The model under review builds one solid part; all positions refer to its coordinate system, in mm. A direction names the side the tool comes from. Round coordinates to 2 decimals unless told otherwise and drop trailing zeros. Write each loop counter-clockwise with the first axis right and the second up, starting at its lowest first coordinate (ties: lowest second). Pieces come first, ordered by that corner, then holes. Notation, with made-up numbers: (42, 68) -> (53, 68) arc R19 cw to (53, 76) -> close; hole circle Ø7 at (-16, -32). An arc over 180 degrees is marked (long way). Answer as a JSON object with one key per item and string values. Group by question number.
1) Mouldability with a two-part tool opening along Z and no side actions: class faces 6 (the flat face through (-20.5, -6, -12)), 7 (the flat face through (-17.458, -7.317, -13.875)), 8 (the flat face through (-17.458, -7.283, -9.545)) as pulls with the +Z half, pulls with the -Z half, needs draft (parallel to the pull), parting line crosses it, or undercut.
2) We need section B-B, the plane x = -17. Write out the cut boundary in (y, z).
3) We need section D-D, the plane x = -8. Write out the cut boundary in (y, z).
4) We need section C-C, the plane z = 7. Write out the cut boundary in (x, y).
5) To check wall thickness, follow probe 1 along X at (y, z) = (-9.5, -5); probe 2 along X at (y, z) = (-8.5, -8); probe 3 along Y at (x, z) = (8, 7.5). State the ranges of each line that lie inside material, in increasing order. Write a range as [from, to].
6) We need section A-A, the plane y = -1. Write out the cut boundary in (x, z).
7) Insertion check: pin 1 Ø1.5 at (y, z) = (3, 3) entering from -X; pin 2 Ø2.5 at (x, z) = (-17, 11.5) entering from +Y; pin 3 Ø5 at (y, z) = (-11.5, -1) entering from -X; pin 4 Ø1.5 at (y, z) = (-6.5, -12.5) entering from -X. Each pin has a flat end and moves straight along its axis. Give the tip position at first contact, or say it passes through.
8) Machinability: for faces 1 (the flat face through (-18, -10.2, 0)), 2 (the flat face through (0, 3, -10.5)), 3 (the flat face through (-17, -8.55, -12)), 4 (the flat face through (-12.1, -6, 0)), 5 (the flat face through (-17, -3.55, -12)), which of the approach directions +Z, -Z, +X, -X, +Y, -Y give a long, thin tool a straight path to every point of the face, cutting with its end or side? Answer none if there is none.
Autodesk Inventor part; units mm, degrees
ref_plane "YZ Plane" through (0, 0, 0) normal (1, 0, 0) x (0, 1, 0)
ref_plane "XZ Plane" through (0, 0, 0) normal (0, 1, 0) x (-1, 0, 0)
ref_plane "XY Plane" through (0, 0, 0) normal (0, 0, 1) x (1, 0, 0)
sketch "Sketch1" plane through (0, 0, 0) normal (0, 1, 0) x (-1, 0, 0)
  line L0 (14.5, -15.5) -> (-14.5, -15.5)
  line L1 (-14.5, -15.5) -> (-14.5, 15.5)
  line L2 (-14.5, 15.5) -> (14.5, 15.5)
  line L3 (14.5, 15.5) -> (14.5, -15.5)
  line L4 (14.5, -15.5) -> (-14.5, 15.5) construction
  line L5 (-14.5, -15.5) -> (14.5, 15.5) construction
  point P0 (0, 0)
  dimension "d0" = 29
  dimension "d1" = 31
extrude "Extrusion1" add sketch "Sketch1" along normal blind 1.6
sketch "Sketch2" plane through (0, 0, 0) normal (0, -1, 0) x (1, 0, 0)
  line L0 (-14.5, 15.5) -> (-12.1, 15.5)
  line L1 (-12.1, 15.5) -> (-12.1, -15.5)
  line L2 (-12.1, -15.5) -> (-14.5, -15.5)
  line L3 (-14.5, -15.5) -> (-14.5, 15.5)
  point P0 (0, 0)
  dimension "d4" = 2.4
extrude "Extrusion2" add sketch "Sketch2" along normal blind 12.8
sketch "Sketch3" plane through (0, 0, 0) normal (0, -1, 0) x (1, 0, 0)
  line L0 (-14.5, 15.5) -> (14.5, 15.5) construction
  line L1 (12.125, 15.5) -> (12.125, -15.5904) construction
  line L2 (14.5, -15.5) -> (14.5, 15.5) construction
  line L3 (12.125, 12.375) -> (14.5, 12.375) construction
  line L4 (12.125, -12.375) -> (14.5, -12.375) construction
  line L5 (-12.1, -15.5) -> (14.5, -15.5) construction
  circle A0 centre (12.125, 12.375) radius 1.625
  circle A1 centre (12.125, -12.375) radius 1.625
  point P0 (0, 0)
  dimension "d7" = 2.375
  dimension "d8" = 3.125
  dimension "d9" = 3.125
  dimension "d10" = 3.25
extrude "Extrusion3" cut sketch "Sketch3" against normal through all
sketch "Sketch4" plane through (-14.5, 1.6, -15.5) normal (-1, 0, 0) x (0, 0, 1)
  line L0 (30.9539, -7.65) -> (0, -7.65) construction
  line L1 (0, -14.4) -> (0, 0) construction
  line L2 (0, 0) -> (31, 0) construction
  line L3 (24.3332, -7.65) -> (25.7766, -5.15)
  line L4 (25.7766, -5.15) -> (28.6634, -5.15)
  line L5 (28.6634, -5.15) -> (30.1068, -7.65)
  line L6 (30.1068, -7.65) -> (28.6634, -10.15)
  line L7 (28.6634, -10.15) -> (25.7766, -10.15)
  line L8 (25.7766, -10.15) -> (24.3332, -7.65)
  line L9 (2.3366, -10.15) -> (0.8932, -7.65)
  line L10 (0.8932, -7.65) -> (2.3366, -5.15)
  line L11 (2.3366, -5.15) -> (5.2234, -5.15)
  line L12 (5.2234, -5.15) -> (6.6668, -7.65)
  line L13 (6.6668, -7.65) -> (5.2234, -10.15)
  line L14 (5.2234, -10.15) -> (2.3366, -10.15)
  line L15 (31, 0) -> (31, -14.4)
  point P0 (15.5, -1.6)
  point P1 (27.22, -7.65)
  point P2 (3.78, -7.65)
  dimension "d13" = 7.65
  dimension "d14" = 5
  dimension "d15" = 3.78
  dimension "d16" = 3.78
extrude "Extrusion4" add sketch "Sketch4" along normal blind 6
sketch "Sketch5" plane through (-14.5, 1.6, -15.5) normal (-1, 0, 0) x (0, 0, 1)
  line L0 (0, 0) -> (31, 0) construction
  line L1 (15.5, 0) -> (15.5, -14.4) construction
  line L2 (31, -14.4) -> (0, -14.4) construction
  line L3 (23.75, -3.8) -> (7.25, -3.8)
  line L4 (7.25, -3.8) -> (7.25, -11.8)
  line L5 (7.25, -11.8) -> (23.75, -11.8)
  line L6 (23.75, -11.8) -> (23.75, -3.8)
  line L7 (23.75, -3.8) -> (7.25, -11.8) construction
  line L8 (7.25, -3.8) -> (23.75, -11.8) construction
  point P0 (15.5, -1.6)
  point P1 (15.5, -7.8)
  dimension "d19" = 3.8
  dimension "d20" = 8
  dimension "d21" = 16.5
extrude "Extrusion5" add sketch "Sketch5" along normal blind 8
sketch "Sketch6" plane through (0, 1.6, 0) normal (0, 1, 0) x (1, 0, 0)
  line L0 (9.5, -10.5) -> (9.5, 10.5)
  line L1 (9.5, 10.5) -> (-9.5, 10.5)
  line L2 (-9.5, 10.5) -> (-9.5, -10.5)
  line L3 (-9.5, -10.5) -> (9.5, -10.5)
  line L4 (9.5, -10.5) -> (-9.5, 10.5) construction
  line L5 (9.5, 10.5) -> (-9.5, -10.5) construction
  line L6 (14.5, -15.5) -> (14.5, 15.5)
  line L7 (-14.5, -15.5) -> (14.5, -15.5)
  point P0 (0, 0)
  dimension "d24" = 5
  dimension "d25" = 5
extrude "Extrusion6" add sketch "Sketch6" along normal blind 3
sketch "Sketch7" plane through (0, 0, 0) normal (0, -1, 0) x (1, 0, 0)
  line L0 (-12.1, 15.5) -> (-12.1, -15.5) construction
  line L1 (-12.1, 0) -> (14.5, 0) construction
  line L2 (14.5, 15.5) -> (14.5, -15.5) construction
  line L3 (14.5, -5.15) -> (14.5, 5.15)
  line L4 (14.5, 5.15) -> (11.8, 5.15)
  line L5 (11.8, 5.15) -> (11.8, -5.15)
  line L6 (11.8, -5.15) -> (14.5, -5.15)
  line L7 (14.5, -5.15) -> (11.8, 5.15) construction
  line L8 (14.5, 5.15) -> (11.8, -5.15) construction
  point P0 (0, 0)
  point P1 (13.15, 0)
  dimension "d28" = 10.3
  dimension "d29" = 2.7
  dimension "d30" = 0
extrude "Extrusion7" add sketch "Sketch7" along normal blind 17
properties part number "RS 232 Board"
Here are the results:
{
 "1": {"face 6": "needs draft", "face 7": "pulls with the -Z half", "face 8": "undercut"},
 "2": {"outline": "(-10.2, -8.25) -> (-2.2, -8.25) -> (-2.2, 8.25) -> (-10.2, 8.25) -> close; (-8.55, -13.16) -> (-6.05, -14.61) -> (-3.55, -13.16) -> (-3.55, -10.28) -> (-6.05, -8.83) -> (-8.55, -10.28) -> close; (-8.55, 10.28) -> (-6.05, 8.83) -> (-3.55, 10.28) -> (-3.55, 13.16) -> (-6.05, 14.61) -> (-8.55, 13.16) -> close"},
 "3": {"outline": "(0, -15.5) -> (1.6, -15.5) -> (1.6, -10.5) -> (4.6, -10.5) -> (4.6, 10.5) -> (1.6, 10.5) -> (1.6, 15.5) -> (0, 15.5) -> close"},
 "4": {"outline": "(-22.5, -10.2) -> (-14.5, -10.2) -> (-14.5, -12.8) -> (-12.1, -12.8) -> (-12.1, 0) -> (14.5, 0) -> (14.5, 1.6) -> (9.5, 1.6) -> (9.5, 4.6) -> (-9.5, 4.6) -> (-9.5, 1.6) -> (-14.5, 1.6) -> (-14.5, -2.2) -> (-22.5, -2.2) -> close"},
 "5": {"probe 1": "x = [-22.5, -12.1], [11.8, 14.5]", "probe 2": "x = [-22.5, -12.1]", "probe 3": "y = [0, 4.6]"},
 "6": {"outline": "(-14.5, -15.5) -> (-12.1, -15.5) -> (-12.1, 15.5) -> (-14.5, 15.5) -> close; (11.8, -5.15) -> (14.5, -5.15) -> (14.5, 5.15) -> (11.8, 5.15) -> close"},
 "7": {"pin 1": "stops at x = -9.5", "pin 2": "stops at y = -3.55", "pin 3": "stops at x = -22.5", "pin 4": "stops at x = -20.5"},
 "8": {"face 1": "+Z, -Z, -X, -Y", "face 2": "-Z, +X, -X, +Y", "face 3": "-Z, -X, -Y", "face 4": "+Z, -Z, -Y", "face 5": "-Z, -X, +Y"}
}
